from build123d import *

# Parameters (mm, degrees)
SKETCH2_R           = 3.75
SKETCH2_R_2         = 1.5
BOSS_EXTRUDE1_DEPTH = 3


with BuildPart() as part:
    # Sketch2 → Boss-Extrude1 (new body)
    # profile 1 of 3: a face of its own
    with BuildSketch(Plane.XY):
        Circle(SKETCH2_R)
        Circle(SKETCH2_R_2, mode=Mode.SUBTRACT)
    # profile 2 of 3: a face of its own
    with BuildSketch(Plane.XY):
        with BuildLine():
            ThreePointArc((3.75, 0), (2.651650429, -2.651650429), (0, -3.75))
            Line((0, -3.75), (100, -3.75))
            ThreePointArc((100, -3.75), (96.25, 0), (100, 3.75))
            Line((100, 3.75), (0, 3.75))
            ThreePointArc((0, 3.75), (2.651650429, 2.651650429), (3.75, 0))
        make_face()
    # profile 3 of 3: a face of its own
    with BuildSketch(Plane.XY):
        with Locations((100, 0)):
            Circle(SKETCH2_R)
        with Locations((100, 0)):
            Circle(SKETCH2_R_2, mode=Mode.SUBTRACT)
    extrude(amount=BOSS_EXTRUDE1_DEPTH)


solid = part.part
Model file for the job. Use its own axes, mm. Round coordinates to 2 decimals unless told otherwise and drop trailing zeros. Loops run counter-clockwise (first coordinate to the right, second up) from the corner with the lowest first, then second, coordinate; pieces in that order, holes last.
1. Band-saw the part on B-B, the plane z = 2.2. List the corners of the cut face in (x, y), and give its area (3 significant figures).
Check values:
outline: (0, -3.75) - (100, -3.75) arc R3.75 ccw to (100, 3.75) - (0, 3.75) arc R3.75 ccw to start; hole circle Ø3 at (0, 0); hole circle Ø3 at (100, 0)
area: 780 mm2
2. Wall check: probe 1 along X at (y, z) = (0.5, 2.6); probe 2 along X at (y, z) = (-0.25, 0.75); probe 3 along Y at (x, z) = (100, 1.8). Give the ranges that are in metal, low to high.
Check values:
probe 1: x = -3.72 to -1.41, 1.41 to 98.59, 101.41 to 103.72
probe 2: x = -3.74 to -1.48, 1.48 to 98.52, 101.48 to 103.74
probe 3: y = -3.75 to -1.5, 1.5 to 3.75
3. Band-saw the part on A-A, the plane y = 0. List the corners of the cut face in (x, z).
Check values:
outline: (-3.75, 0) - (-1.5, 0) - (-1.5, 3) - (-3.75, 3) - close; (1.5, 0) - (98.5, 0) - (98.5, 3) - (1.5, 3) - close; (101.5, 0) - (103.75, 0) - (103.75, 3) - (101.5, 3) - close
4. Drop a flat-ended pin along its axis: P1, Ø1, axis at y = 2, z = 1, coming from the -X side. Give the stop position or say it passes through.
Check values:
P1: stops at x = -3.44
5. Mould opens along Y. For faces 1 (the flat face through (49, -3.75, 1)), 2 (the cylindrical face through (103.75, -0.08, 1.48)), 3 (the cylindrical face through (100.806, 1.265, 1.479)) say: +Y half, -Y half, draft (parallel to the pull), parting line (faces both ways), or undercut.
Check values:
face 1: -Y half
face 2: parting line
face 3: undercut
